from build123d import *

# Parameters (mm, degrees)
SKETCH_1_R        = 3
SKETCH_1_R_2      = 1.5
EXTRUDE_1_DEPTH   = 3
EXTRUDE_1_2_DEPTH = 3
SKETCH_2_R        = 1.5
EXTRUDE_2_DEPTH   = 129.8
SKETCH_3_R        = 3
SKETCH_3_R_2      = 1.5
EXTRUDE_3_DEPTH   = 1.5
SKETCH_4_R        = 3
SKETCH_4_R_2      = 1.5
EXTRUDE_4_DEPTH   = 1.4


with BuildPart() as part:
    # Sketch 1 → Extrude 1 (new body)
    with BuildSketch(Plane(origin=(0, 0, 0), x_dir=(1, 0, 0), z_dir=(0, 1, 0))):
        Circle(SKETCH_1_R)
        Circle(SKETCH_1_R_2, mode=Mode.SUBTRACT)
    extrude(amount=EXTRUDE_1_DEPTH)



with BuildPart() as body_2:
    # Sketch 1 → Extrude 1 2 (new body)
    with BuildSketch(Plane(origin=(0, 0, 0), x_dir=(1, 0, 0), z_dir=(0, 1, 0))):
        with Locations((0, -133)):
            Circle(SKETCH_1_R)
        with Locations((0, -133)):
            Circle(SKETCH_1_R_2, mode=Mode.SUBTRACT)
    extrude(amount=EXTRUDE_1_2_DEPTH)


with BuildPart() as part_1:
    add(part.part)

    add(body_2.part)  # Extrude 2 merges body 2
    # Sketch 2 → Extrude 2 (add)
    with BuildSketch(Plane.XY.offset(1.6)):
        with Locations((0, 1.5)):
            Circle(SKETCH_2_R)
    extrude(amount=EXTRUDE_2_DEPTH)

    # Sketch 3 → Extrude 3 (add)
    with BuildSketch(Plane(origin=(0, 3, 0), x_dir=(1, 0, 0), z_dir=(0, 1, 0))):
        Circle(SKETCH_3_R)
        Circle(SKETCH_3_R_2, mode=Mode.SUBTRACT)
    extrude(amount=EXTRUDE_3_DEPTH)

    # Sketch 4 → Extrude 4 (add)
    with BuildSketch(Plane(origin=(0, 3, 0), x_dir=(1, 0, 0), z_dir=(0, 1, 0))):
        with Locations((0, -133)):
            Circle(SKETCH_4_R)
        with Locations((0, -133)):
            Circle(SKETCH_4_R_2, mode=Mode.SUBTRACT)
    extrude(amount=EXTRUDE_4_DEPTH)


solid = part_1.part
Model file for the job. Use its own axes, mm. A direction names the side the tool comes from. Give positions to 0.01 mm unless a question says otherwise; leave off trailing zeros. Order: outer loops, then holes, each group sorted by start corner. A loop starts at its lowest first (then second) coordinate and runs counter-clockwise, first axis right, second up. Notation, with made-up numbers: M 35,-28.5 L 45,-28.5 A25 cw 45,1.5 Z; hole C -26.75,64.5 d8. An arc over 180 degrees is marked long. Write item = value, one per line.
Q1. Cut at A-A, the plane z = 0. List the corners of the cut face in (x, y), then the cut area to 3 significant figures.
Derived:
outline = M -3,0 L -1.5,0 L -1.5,4.5 L -3,4.5 Z; M 1.5,0 L 3,0 L 3,4.5 L 1.5,4.5 Z
area = 13.5 mm2
Q2. Tool access for faces 1 (the flat face through (1.3, 4.4, 134.3)), 2 (the flat face through (1.3, 0, 1.3)): list every direction of +Z, -Z, +X, -X, +Y, -Y with a clear straight run to the whole face (end or side of a thin tool).
Derived:
face_1 = +Z, +X, -X, +Y
face_2 = +Z, -Z, +X, -X, -Y
Q3. Cut at C-C, the plane z = 133. List the corners of the cut face in (x, y), then the cut area to 3 significant figures.
Derived:
outline = M -3,0 L -1.5,0 L -1.5,4.4 L -3,4.4 Z; M 1.5,0 L 3,0 L 3,4.4 L 1.5,4.4 Z
area = 13.2 mm2
Q4. Cut at D-D, the plane z = 119. List the corners of the cut face in (x, y), then the cut area to 3 significant figures.
Derived:
outline = C 0,1.5 d3
area = 7.07 mm2
Q5. Cut at B-B, the plane y = 1.5. List the corners of the cut face in (x, z).
Derived:
outline = M -1.5,2.6 A3 ccw long 1.5,2.6 L 1.5,130.4 A3 ccw long -1.5,130.4 Z; hole C 0,0 d3; hole C 0,133 d3
Q6. Drill centre lines: line 1 (Z direction, x = 0, y = 2.3); line 2 (Z direction, x = 1.25, y = 3.1); line 3 (X direction, y = 1.3, z = 0). Where is each one in solid material? Low to high. Write a range as [from, to].
Derived:
line_1 = [-3, -1.5], [1.5, 131.5], [134.5, 136]
line_2 = [-2.73, -0.83], [0.83, 2.73], [130.27, 132.17], [133.83, 135.73]
line_3 = [-3, -1.5], [1.5, 3]
Q7. Flat gauge pins, fed straight in: pin 1 (1.5 mm diameter, centred on x = -2, z = 82, fed in from +Y); pin 2 (1.8 mm diameter, centred on x = -1, z = 131.5, fed in from +Y). Where does each tip first touch, or does it go through?
Derived:
pin_1 = 2.33
pin_2 = 4.4
Q8. Two-plate mould, pull along X, no slides. Class faces 3 (the flat face through (1.3, 4.5, 1.3)), 4 (the cylindrical face through (-0.195, 2.169, 131.513)), 5 (the cylindrical face through (-1.11, 2.51, 65.61)): pulls with the +X half, pulls with the -X half, needs draft (parallel to the pull), parting line crosses it, or undercut.
Derived:
face_3 = needs draft
face_4 = undercut
face_5 = parting line crosses it
